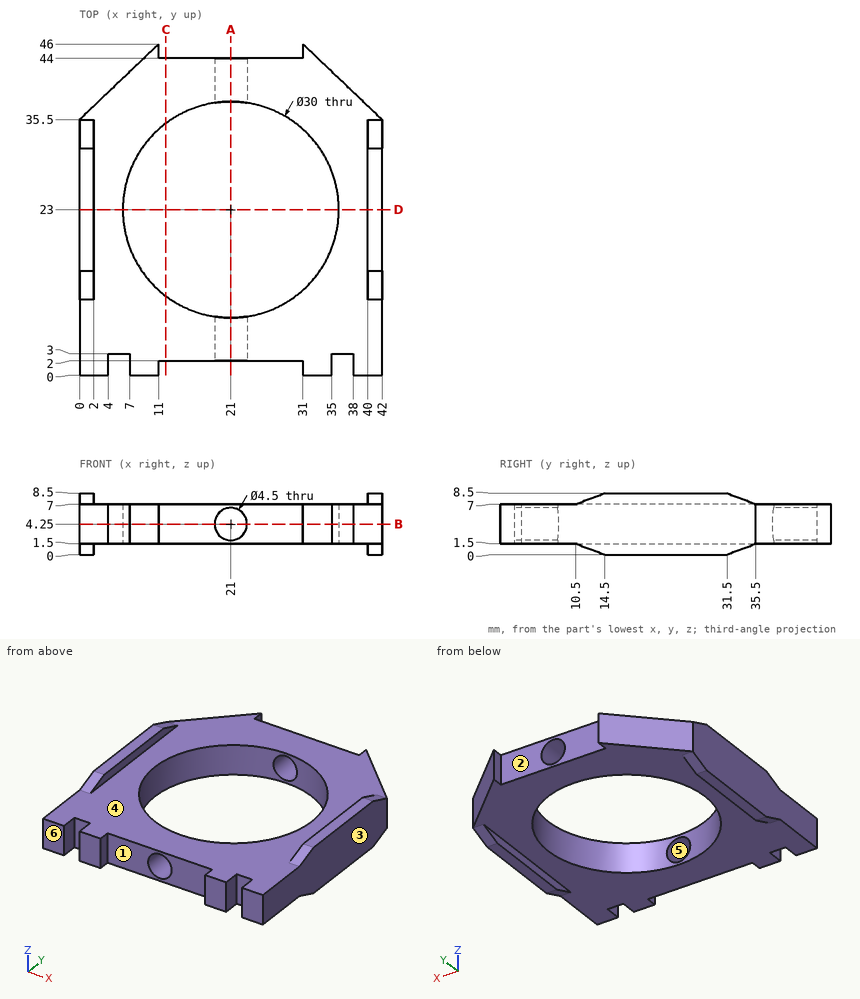
Geometry check sheet. Reference: drawing and pictorial views, mm from the part's lowest x, y, z. A direction names the side the tool comes from. Round coordinates to 2 decimals unless told otherwise and drop trailing zeros. Loops run counter-clockwise (first coordinate to the right, second up) from the corner with the lowest first, then second, coordinate; pieces in that order, holes last. Notation, with made-up numbers: M -12,22 L 18,22 A20 cw 18,61 Z; hole C 63.25,47 d10. An arc over 180 degrees is marked long. Return JSON: item names as keys, results as strings. Group by question number.
(1) Mould release check, pull along Z, two halves, no side actions. Record for the marked faces 4, 5 and 6: pulls with the +Z half, pulls with the -Z half, needs draft (parallel to the pull), parting line crosses it, or undercut.
(2) Section check A-A, the plane x = 21. Enter the section's corners in (y, z).
(3) Section check D-D, the plane y = 23. Enter the section's corners in (x, z), and give its area (3 significant figures).
(4) Scan lines: line 1 along Z through (x, y) = (21, 40.5); line 2 along X through (y, z) = (14, 7.25); line 3 along Z through (x, y) = (11, 3). Record each from-to range of solid material in increasing order. Write a range as [from, to].
(5) Section check B-B, the plane z = 4.25. Enter the section's corners in (x, y).
(6) Section check C-C, the plane x = 12. Enter the section's corners in (y, z), and give its area (3 significant figures).
(7) Go/stop test with flat-tipped pins: pin 1 (1 mm diameter, centred on x = 34, y = 7, fed in from +Z); pin 2 (4 mm diameter, centred on x = 7, z = 2, fed in from +Y); pin 3 (1 mm diameter, centred on y = 45, z = 5.5, fed in from +X). Record where each tip stops, or that it passes through.
(8) Set-up check for the marked faces 1, 2 and 3: record each of +Z, -Z, +X, -X, +Y, -Y from which the full face is reachable in a straight line by a thin tool's end or side.
Data:
{
 "1": {"face 4": "pulls with the +Z half", "face 5": "undercut", "face 6": "needs draft"},
 "2": {"outline": "M 2,1.5 L 8,1.5 L 8,2 L 2,2 Z; M 2,6.5 L 8,6.5 L 8,7 L 2,7 Z; M 38,1.5 L 44,1.5 L 44,2 L 38,2 Z; M 38,6.5 L 44,6.5 L 44,7 L 38,7 Z"},
 "3": {"outline": "M 0,0 L 2,0 L 2,1.5 L 6,1.5 L 6,7 L 2,7 L 2,8.5 L 0,8.5 Z; M 36,1.5 L 40,1.5 L 40,0 L 42,0 L 42,8.5 L 40,8.5 L 40,7 L 36,7 Z", "area": "78.0 mm²"},
 "4": {"line 1": "[1.5, 2], [6.5, 7]", "line 2": "[0, 2], [40, 42]", "line 3": "[1.5, 7]"},
 "5": {"outline": "M 0,0 L 4,0 L 4,3 L 7,3 L 7,0 L 11,0 L 11,2 L 18.75,2 L 18.75,8.17 A15 cw 18.75,37.83 L 18.75,44 L 11,44 L 11,46 L 0,35.5 Z; M 23.25,2 L 31,2 L 31,0 L 35,0 L 35,3 L 38,3 L 38,0 L 42,0 L 42,35.5 L 31,46 L 31,44 L 23.25,44 L 23.25,37.83 A15 cw 23.25,8.17 Z"},
 "6": {"outline": "M 2,1.5 L 11,1.5 L 11,7 L 2,7 Z; M 35,1.5 L 44,1.5 L 44,7 L 35,7 Z", "area": "99.0 mm²"},
 "7": {"pin 1": "z = 7", "pin 2": "y = 44.09", "pin 3": "x = 32.57"},
 "8": {"face 1": "+Z, -Z, -Y", "face 2": "+Z, -Z, +Y", "face 3": "+Z, -Z, +X, +Y, -Y"}
}
